Print and shaded views of the part. All mm, measured from the part's lowest x, y and z. Round coordinates to 2 decimals unless told otherwise and drop trailing zeros. Loops run counter-clockwise (first coordinate to the right, second up) from the corner with the lowest first, then second, coordinate; pieces in that order, holes last. Notation, with made-up numbers: (31.25, 75.5) -> (78.25, 75.5) arc R27 ccw to (78.25, 112.5) -> close; hole circle Ø10 at (82.5, 10.25). An arc over 180 degrees is marked (long way). Answer as CSV lines item,"result".
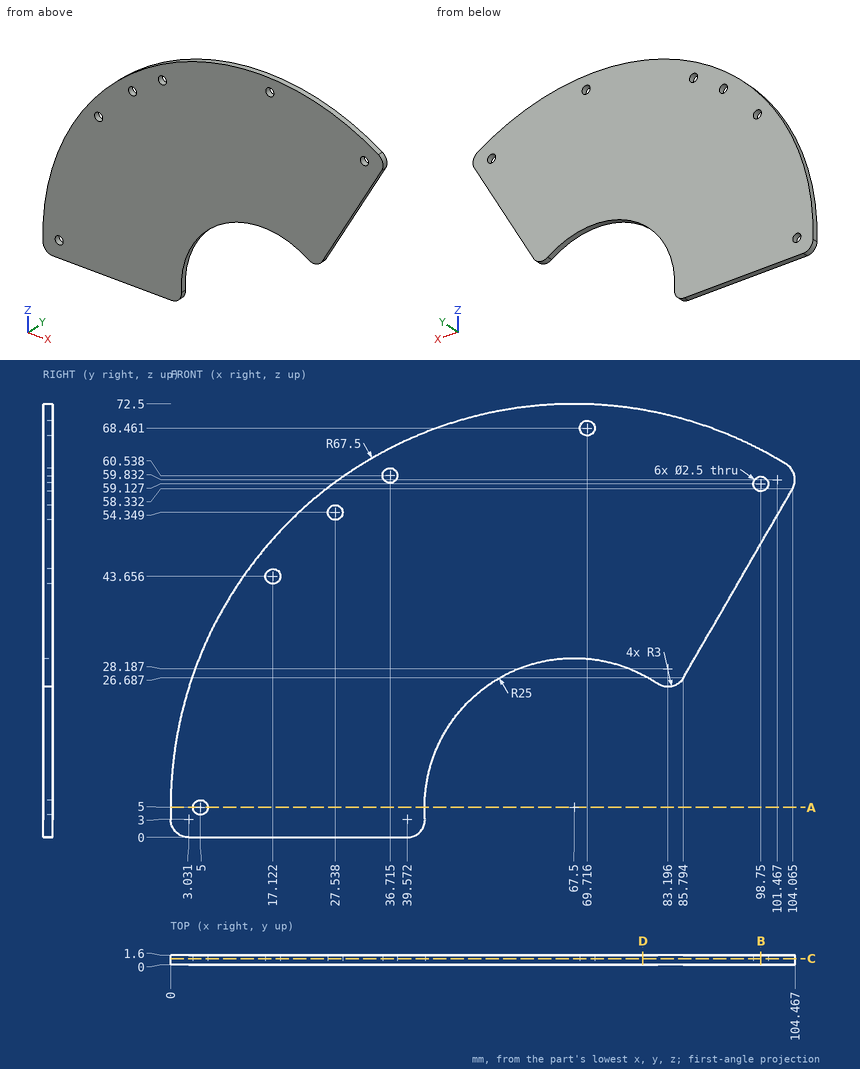
Q1. Saw through at B-B, the plane x = 98.75. Write the cut outline in (y, z).
Geometry results:
outline,"(0, 49.13) -> (1.6, 49.13) -> (1.6, 57.88) -> (0, 57.88) -> close; (0, 60.38) -> (1.6, 60.38) -> (1.6, 64.83) -> (0, 64.83) -> close"
Q2. Saw through at C-C, the plane y = 1.05. Give the number of separate pieces and of enclosed holes in the cut face, then the cut area to 4 significant figures.
Geometry results:
separate pieces,"1"
enclosed holes,"6"
area,"4,505 mm2"
Q3. Drill centre lines: line 1 along X through (y, z) = (1.3, 5); line 2 along X through (y, z) = (1, 43) (1 decimal); line 3 along Z through (x, y) = (74, 1.2) (1 decimal). Where is each one in solid material? Low to high.
Geometry results:
line 1,"0 to 3.75, 6.25 to 42.5"
line 2,"11.7 to 16.1, 18.2 to 95.2"
line 3,"29.1 to 72.2"
Q4. Saw through at A-A, the plane z = 5. Write the cut outline in (x, y).
Geometry results:
outline,"(0, 0) -> (3.75, 0) -> (3.75, 1.6) -> (0, 1.6) -> close; (6.25, 0) -> (42.5, 0) -> (42.5, 1.6) -> (6.25, 1.6) -> close"
Q5. Saw through at D-D, the plane x = 79. Write the cut outline in (y, z).
Geometry results:
outline,"(0, 27.2) -> (1.6, 27.2) -> (1.6, 71.51) -> (0, 71.51) -> close"
Q6. Drop flat-ended pins along their axis: P1, Ø4, axis at x = 36.71, z = 60.54, coming from the -Y side; P2, Ø2, axis at x = 69.72, z = 68.46, coming from the -Y side. Give the stop position or say it passes through.
Geometry results:
P1,"y = 0"
P2,"through"
